Input: part model. Units: mm. Frame: model coordinates. Round coordinates to 2 decimals unless told otherwise and drop trailing zeros. Order: outer loops, then holes, each group sorted by start corner. A loop starts at its lowest first (then second) coordinate and runs counter-clockwise, first axis right, second up. Notation, with made-up numbers: (39, 19) - (47, 19) arc R24 cw to (47, 54) - close; hole circle Ø11 at (-2.75, 27.25). An arc over 180 degrees is marked (long way). One line per item, written item: value. Start each with the question number.
Autodesk Inventor part; units mm, degrees
ref_plane "YZ Plane" through (0, 0, 0) normal (1, 0, 0) x (0, 1, 0)
ref_plane "XZ Plane" through (0, 0, 0) normal (0, 1, 0) x (-1, 0, 0)
ref_plane "XY Plane" through (0, 0, 0) normal (0, 0, 1) x (1, 0, 0)
sketch "Sketch1" plane through (0, 0, 0) normal (0, 0, 1) x (1, 0, 0)
  line L0 (0, 0) -> (293.4944, 0) construction
  line L1 (293.4944, 0) -> (293.4944, -132.0217) construction
  line L2 (293.4944, -132.0217) -> (0, -132.0217) construction
  line L3 (0, -132.0217) -> (0, 0) construction
  line L4 (79.3681, -56.3049) -> (159.3681, -56.3049) construction
  line L5 (283.1562, -93.1287) -> (274.2161, -88.6482) construction
  line L6 (283.1562, -93.1287) -> (282.3201, -93.1287) construction
  line L7 (18.3483, -97.5091) -> (27.4302, -93.3236) construction
  line L8 (18.3483, -97.5091) -> (20.5956, -97.5091) construction
  arc A0 (103.0994, -81.9859) -> (27.4302, -93.3236) centre (93.4367, -275.677) ccw
  arc A1 (274.2161, -88.6482) -> (204.4098, -79.893) centre (217.7822, -255.937) ccw
  arc A2 (103.0994, -81.9859) -> (204.4098, -79.893) centre (140.8276, 544.7964) ccw
  line L9 (27.4302, -93.3236) -> (27.4302, -72.2735)
  line L10 (27.4302, -72.2735) -> (272.6166, -67.591)
  line L11 (272.6166, -67.591) -> (274.2161, -88.6482)
  line L12 (103.0994, -81.9859) -> (86.3195, -71.1488) construction
  line L13 (204.4098, -79.893) -> (220.9707, -68.5773) construction
  line L14 (86.3195, -71.1488) -> (86.3195, -81.1488) construction
  line L15 (86.3195, -81.1488) -> (103.0994, -81.9859) construction
  line L16 (220.9707, -68.5773) -> (221.7303, -78.5773) construction
  line L17 (221.7303, -78.5773) -> (204.4098, -79.893) construction
  dimension "d5" = 80
  dimension "d85" = 10
  dimension "d87" = 26.619
  dimension "d92" = 10
  dimension "d94" = 24.743
  dimension "d100" = 22.985
  dimension "d101" = 22.755
  dimension "d106" = 10
  dimension "d111" = 10
  dimension "d112" = 30
  dimension "d113" = 30
extrude "Extrusion1" add sketch "Sketch1" along normal blind 10
sketch "Sketch2" plane through (0, 0, 10) normal (0, 0, 1) x (1, 0, 0)
  arc A0 (103.0994, -81.9859) -> (204.4098, -79.893) centre (140.8276, 544.7964) ccw
  line L0 (272.6166, -67.591) -> (27.4302, -72.2735)
  line L1 (27.4302, -72.2735) -> (27.4302, -93.3236)
  line L2 (274.2161, -88.6482) -> (272.6166, -67.591)
  line L3 (125.3768, -83.1204) -> (158.7723, -83.1204)
  line L4 (140.8276, -83.1204) -> (140.8276, -70.1078)
  line L5 (140.8276, -76.6141) -> (27.4302, -76.6141)
  line L6 (140.8276, -76.6141) -> (273.302, -76.6141)
  arc A1 (274.2161, -88.6482) -> (204.4098, -79.893) centre (217.7822, -255.937) ccw
  line L7 (274.2161, -88.6482) -> (272.6166, -67.591)
  line L8 (272.6166, -67.591) -> (27.4302, -72.2735)
  line L9 (27.4302, -72.2735) -> (27.4302, -93.3236)
  arc A2 (103.0994, -81.9859) -> (27.4302, -93.3236) centre (93.4367, -275.677) ccw
  arc A3 (103.0994, -81.9859) -> (204.4098, -79.893) centre (140.8276, 544.7964) ccw
  line L10 (140.8276, -83.1204) -> (140.4575, -63.7401)
  point P0 (0, 0)
  point P1 (204.4098, -79.893)
  point P2 (140.5792, -70.1126)
  point P3 (140.7034, -76.6141)
  dimension "d121" = 113.3974
  dimension "d122" = 132.4743
extrude "Extrusion2" cut sketch "Sketch2" against normal blind 10 contours L4 L6 L2 A1 A0 | L10 L5 L4 | L5 L10 L0 L4 | L4 L0 L2 L6
sketch "Sketch4" plane through (0, 0, 10) normal (0, 0, 1) x (1, 0, 0)
  line L0 (140.5792, -70.1126) -> (27.4302, -72.2735)
  line L1 (27.4302, -72.2735) -> (27.4302, -93.3236)
  arc A0 (103.0994, -81.9859) -> (27.4302, -93.3236) centre (93.4367, -275.677) ccw
  arc A1 (103.0994, -81.9859) -> (140.8276, -83.1204) centre (140.8276, 544.7964) ccw
  line L2 (27.4302, -72.2735) -> (27.4302, -93.3236)
  arc A2 (103.0994, -81.9859) -> (27.4302, -93.3236) centre (93.4367, -275.677) ccw
  line L3 (27.4302, -72.2735) -> (27.8295, -93.1796)
  line L4 (140.8276, -83.1204) -> (140.5792, -70.1126)
  point P0 (0, 0)
  point P1 (253.7282, -67.9517)
  dimension "d128" = 90
extrude "Extrusion4" cut sketch "Sketch4" against normal blind 10 contours L3 A0 L1
sketch "Sketch6" plane through (0, 0, 10) normal (0, 0, 1) x (1, 0, 0)
  line L0 (27.4302, -72.2735) -> (27.8295, -93.1796)
  arc A0 (103.0994, -81.9859) -> (27.8295, -93.1796) centre (93.4367, -275.677) ccw
  arc A1 (103.0994, -81.9859) -> (140.8276, -83.1204) centre (140.8276, 544.7964) ccw
  line L1 (140.8276, -83.1204) -> (140.5792, -70.1126)
  line L2 (140.5792, -70.1126) -> (27.4302, -72.2735)
  line L3 (140.5792, -70.1126) -> (27.4302, -72.2735)
  line L4 (140.5792, -70.1126) -> (154.0767, -69.8548)
  line L5 (154.0767, -69.8548) -> (154.3252, -82.8626)
  line L6 (140.5792, -70.1126) -> (140.8276, -83.1204)
  line L7 (154.3252, -82.8626) -> (140.8276, -83.1204)
  point P0 (0, 0)
  dimension "d131" = 13.5
  dimension "d132" = 0
  dimension "d135" = 180
extrude "Extrusion5" add sketch "Sketch6" against normal blind 10 contours L4 L5 L7 L1
sketch "Sketch7" plane through (0, 0, 10) normal (0, 0, 1) x (1, 0, 0)
  line L0 (27.4302, -72.2735) -> (27.8295, -93.1796)
  arc A0 (103.0994, -81.9859) -> (27.8295, -93.1796) centre (93.4367, -275.677) ccw
  arc A1 (103.0994, -81.9859) -> (140.8276, -83.1204) centre (140.8276, 544.7964) ccw
  line L1 (140.8276, -83.1204) -> (154.3252, -82.8626)
  line L2 (154.3252, -82.8626) -> (154.0767, -69.8548)
  line L3 (154.0767, -69.8548) -> (27.4302, -72.2735)
  line L4 (280.7233, -67.4361) -> (281.1225, -88.3423)
  arc A2 (281.1225, -88.3423) -> (205.4801, -80.0307) centre (222.5312, -273.2116) ccw
  arc A3 (167.8227, -82.6048) -> (205.4801, -80.0307) centre (143.8479, 544.854) ccw
  line L5 (167.8227, -82.6048) -> (154.3252, -82.8626)
  line L6 (154.0767, -69.8548) -> (280.7233, -67.4361)
  point P0 (0, 0)
extrude "Extrusion6" add sketch "Sketch7" against normal blind 10 contours L6 L4 A2 A3 L5 L2
equation "\"d111\" = d106"
equation "\"d113\" = d112"
properties part number "deseczka_dol_check - 6"
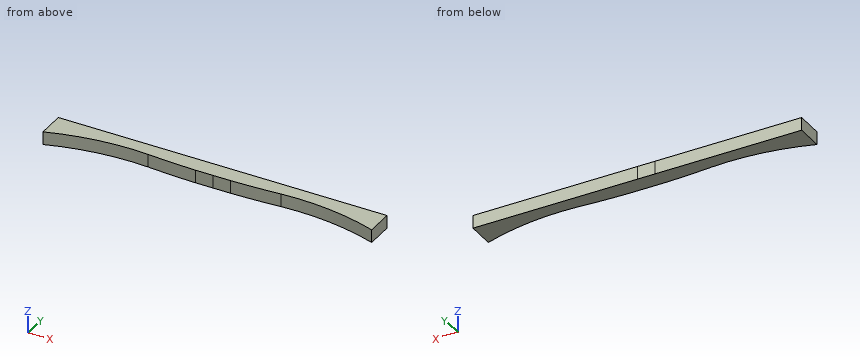
Item 1: First-contact query: pin 1 Ø4 at (y, z) = (-79.5, 6.5) entering from -X; pin 2 Ø6 at (x, y) = (106, -87) entering from +Z. Flat tips, straight axial feed; report the tip coordinate or a pass-through.
Item 2: Section query C-C on x = 226. Return loops of the section in (y, z).
Item 3: Line query: L1, parallel to Y at x = 71, z = 1.5; L2, parallel to Y at x = 174, z = 8.75; L3, parallel to X at y = -73.25, z = 6.75. Output: solid intervals per line, ascending.
Item 4: Section query D-D on x = 156.5. Return loops of the section in (y, z), and give its area (3 significant figures).
Geometry results:
1. pin 1: stops at x = 27.53
1. pin 2: passes through
2. outline: (-79.31, 0) - (-68.48, 0) - (-68.48, 10) - (-79.31, 10) - close
3. L1: y = -83.05 to -71.44
3. L2: y = -82.34 to -69.47
3. L3: x = 27.45 to 280.83
4. outline: (-82.82, 0) - (-69.81, 0) - (-69.81, 10) - (-82.82, 10) - close
4. area: 130 mm^2
